Check sheet for the modelled part. Datum: model origin and axes. Units: mm. A direction names the side the tool comes from. Round coordinates to 2 decimals unless told otherwise and drop trailing zeros. Order: outer loops, then holes, each group sorted by start corner. A loop starts at its lowest first (then second) coordinate and runs counter-clockwise, first axis right, second up.
(1) Tool access check on faces 1 (the cylindrical face through (-42.3, -0.1, 8.5)), 2 (the cylindrical face through (-39.5, -0.1, 6.9)), 3 (the cylindrical face through (-35.14, 0.11, 3.9)), 4 (the flat face through (-1, 7.5, 2)). Record the directions out of +Z, -Z, +X, -X, +Y, -Y that give a thin tool (end or side, any length) a straight path to the whole face; none if there is none.
(2) Sectioned sample at A-A, the plane z = 1.5. Count the separate pieces of the cut face and the enclosed holes in it, and give its area (3 significant figures).
(3) Sectioned sample at C-C, the plane x = -10. Enter the section's corners in (y, z).
(4) Mould release check, pull along Y, two halves, no side actions. Record for faces 5 (the cylindrical face through (35.14, -0.11, 3.9)), 6 (the cylindrical face through (-39.6, 11.6, 6.4)), 7 (the flat face through (37.4, 0, 8)): released by +Y, released by -Y, zero draft, split by the parting line, or undercut.
(5) Thickness scan on probe 1 along Y at (x, z) = (-10, 0.9); probe 2 along X at (y, z) = (4, 2.35); probe 3 along Y at (x, z) = (-39.5, 3.25). Record the ranges inside material, lowest first.
(6) Depth check by flat-ended pin: pin 1 (3 mm diameter, centred on x = -7.5, z = 3.5, fed in from +Y); pin 2 (12 mm diameter, centred on x = -3, y = -2.5, fed in from +Z); pin 3 (2 mm diameter, centred on x = -9.5, z = 3, fed in from -Y). Enter the tip coordinate at first touch or a pass-through.
(7) Sectioned sample at B-B, the plane x = 39.5. Enter the section's corners in (y, z), and give its area (3 significant figures).
```python
from build123d import *

# Parameters (mm, degrees)
SKETCH1_W                                  = 86
SKETCH1_H                                  = 15
BOSS_EXTRUDE1_DEPTH                        = 3
SKETCH2_W                                  = 7
SKETCH2_H                                  = 15
BOSS_EXTRUDE2_DEPTH                        = 10
SKETCH5_R                                  = 4.5
CUT_EXTRUDE1_DEPTH                         = 88.299770905
SKETCH6_R                                  = 6.1
CUT_EXTRUDE4_DEPTH                         = 2.1
BOSS_EXTRUDE3_DEPTH                        = 13
SKETCH8_R                                  = 1.75
CUT_EXTRUDE5_DEPTH                         = 47.395689455
SKETCH9_R                                  = 1.75
CUT_EXTRUDE6_DEPTH                         = 46.6460294
MIRROR1_AT_THE_SECOND_PLANE_COPY_1_SKETC_R = 6.1
MIRROR1_AT_THE_SECOND_PLANE_COPY_1_DEPTH   = 2.1
MIRROR1_AT_THE_SECOND_PLANE_COPY_2_DEPTH   = 13
MIRROR1_AT_THE_SECOND_PLANE_COPY_3_SKETC_R = 1.75
MIRROR1_AT_THE_SECOND_PLANE_COPY_3_DEPTH   = 47.395689455
MIRROR1_AT_THE_SECOND_PLANE_COPY_4_SKETC_R = 1.75
MIRROR1_AT_THE_SECOND_PLANE_COPY_4_DEPTH   = 46.6460294
FILLET1_R                                  = 3


with BuildPart() as part:
    # Sketch1 → Boss-Extrude1 (new body)
    with BuildSketch(Plane.XY):
        Rectangle(SKETCH1_W, SKETCH1_H)
    extrude(amount=BOSS_EXTRUDE1_DEPTH)

    # Sketch2 → Boss-Extrude2 (add)
    with BuildSketch(Plane.XY.offset(3)):
        with Locations((-39.5, 0)):
            Rectangle(SKETCH2_W, SKETCH2_H)
        with Locations((39.5, 0)):
            Rectangle(SKETCH2_W, SKETCH2_H)
    extrude(amount=BOSS_EXTRUDE2_DEPTH)

    # Sketch5 → Cut-Extrude1 (cut, through all)
    with BuildSketch(Plane(origin=(43, 0, 0), x_dir=(0, 0, -1), z_dir=(1, 0, 0))):
        with Locations((-13, 0)):
            Circle(SKETCH5_R)
    extrude(amount=-CUT_EXTRUDE1_DEPTH, mode=Mode.SUBTRACT)

    # Sketch6 → Cut-Extrude4 (cut, symmetric)
    with BuildSketch(Plane(origin=(39.5, 0, 0), x_dir=(0, 0, -1), z_dir=(1, 0, 0))):
        with Locations((-13, 0)):
            Circle(SKETCH6_R)
    cut_extrude4 = extrude(amount=CUT_EXTRUDE4_DEPTH, both=True, mode=Mode.SUBTRACT)

    # Sketch7 → Boss-Extrude3 (add)
    with BuildSketch(Plane.XY):
        with BuildLine():
            Line((37.4, 6.1), (41.6, 6.1))
            Line((41.6, 6.1), (41.6, 4.5))
            Line((41.6, 4.5), (43, 4.5))
            Line((43, 4.5), (43, 8.1))
            ThreePointArc((43, 8.1), (39.5, 11.6), (36, 8.1))
            Line((36, 8.1), (36, 4.5))
            Line((36, 4.5), (37.4, 4.5))
            Line((37.4, 4.5), (37.4, 6.1))
        make_face()
    boss_extrude3 = extrude(amount=BOSS_EXTRUDE3_DEPTH)

    # Sketch8 → Cut-Extrude5 (cut, symmetric)
    with BuildSketch(Plane.XY.offset(13)):
        with Locations((39.5, 8.6)):
            Circle(SKETCH8_R)
    cut_extrude5 = extrude(amount=CUT_EXTRUDE5_DEPTH, both=True, mode=Mode.SUBTRACT)

    # Sketch9 → Cut-Extrude6 (cut, through all)
    with BuildSketch(Plane.XY.offset(3)):
        with Locations((-10, -4)):
            Circle(SKETCH9_R)
    cut_extrude6 = extrude(amount=-CUT_EXTRUDE6_DEPTH, mode=Mode.SUBTRACT)

    # Mirror1: Cut-Extrude4, Boss-Extrude3, Cut-Extrude5, Cut-Extrude6 across plane
    add(cut_extrude4.mirror(Plane(origin=(0, 0, 0), x_dir=(0, 0, 1), z_dir=(1, 0, 0))), mode=Mode.SUBTRACT)
    add(boss_extrude3.mirror(Plane(origin=(0, 0, 0), x_dir=(0, 0, 1), z_dir=(1, 0, 0))))
    add(cut_extrude5.mirror(Plane(origin=(0, 0, 0), x_dir=(0, 0, 1), z_dir=(1, 0, 0))), mode=Mode.SUBTRACT)
    add(cut_extrude6.mirror(Plane(origin=(0, 0, 0), x_dir=(0, 0, 1), z_dir=(1, 0, 0))), mode=Mode.SUBTRACT)

    # Mirror1 at the second plane: Cut-Extrude4, Boss-Extrude3, Cut-Extrude5, Cut-Extrude6 across plane
    add(cut_extrude4.mirror(Plane.ZX), mode=Mode.SUBTRACT)
    add(boss_extrude3.mirror(Plane.ZX))
    add(cut_extrude5.mirror(Plane.ZX), mode=Mode.SUBTRACT)
    add(cut_extrude6.mirror(Plane.ZX), mode=Mode.SUBTRACT)

    # Mirror1 at the second plane copy 1 sketc → Mirror1 at the second plane copy 1 (cut, symmetric)
    with BuildSketch(Plane(origin=(-39.5, 0, 0), x_dir=(0, 0, -1), z_dir=(-1, 0, 0))):
        with Locations((-13, 0)):
            Circle(MIRROR1_AT_THE_SECOND_PLANE_COPY_1_SKETC_R)
    extrude(amount=MIRROR1_AT_THE_SECOND_PLANE_COPY_1_DEPTH, both=True, mode=Mode.SUBTRACT)

    # Mirror1 at the second plane copy 2 sketc → Mirror1 at the second plane copy 2 (add)
    with BuildSketch(Plane(origin=(0, 0, 0), x_dir=(-1, 0, 0), z_dir=(0, 0, 1))):
        with BuildLine():
            Line((37.4, 6.1), (41.6, 6.1))
            Line((41.6, 6.1), (41.6, 4.5))
            Line((41.6, 4.5), (43, 4.5))
            Line((43, 4.5), (43, 8.1))
            ThreePointArc((43, 8.1), (39.5, 11.6), (36, 8.1))
            Line((36, 8.1), (36, 4.5))
            Line((36, 4.5), (37.4, 4.5))
            Line((37.4, 4.5), (37.4, 6.1))
        make_face()
    extrude(amount=MIRROR1_AT_THE_SECOND_PLANE_COPY_2_DEPTH)

    # Mirror1 at the second plane copy 3 sketc → Mirror1 at the second plane copy 3 (cut, symmetric)
    with BuildSketch(Plane(origin=(0, 0, 13), x_dir=(-1, 0, 0), z_dir=(0, 0, 1))):
        with Locations((39.5, 8.6)):
            Circle(MIRROR1_AT_THE_SECOND_PLANE_COPY_3_SKETC_R)
    extrude(amount=MIRROR1_AT_THE_SECOND_PLANE_COPY_3_DEPTH, both=True, mode=Mode.SUBTRACT)

    # Mirror1 at the second plane copy 4 sketc → Mirror1 at the second plane copy 4 (cut, through all)
    with BuildSketch(Plane(origin=(0, 0, 3), x_dir=(-1, 0, 0), z_dir=(0, 0, 1))):
        with Locations((-10, -4)):
            Circle(MIRROR1_AT_THE_SECOND_PLANE_COPY_4_SKETC_R)
    extrude(amount=-MIRROR1_AT_THE_SECOND_PLANE_COPY_4_DEPTH, mode=Mode.SUBTRACT)

    # Fillet1
    fillet1_edges = [part.edges().sort_by_distance(p)[0] for p in [
        (-36, 0, 3),
        (36, 0, 3),
    ]]
    fillet(fillet1_edges, radius=FILLET1_R)


solid = part.part
```
Derived:
1. face 1: +Z, +X, -X
1. face 2: +Z
1. face 3: +Z, +Y, -Y
1. face 4: +Z, -Z, +Y
2. separate pieces: 1
2. enclosed holes: 8
2. area: 1,310 mm2
3. outline: (-7.5, 0) - (-5.75, 0) - (-5.75, 3) - (-7.5, 3) - close; (-2.25, 0) - (2.25, 0) - (2.25, 3) - (-2.25, 3) - close; (5.75, 0) - (7.5, 0) - (7.5, 3) - (5.75, 3) - close
4. face 5: zero draft
4. face 6: released by +Y
4. face 7: undercut
5. probe 1: y = -7.5 to -5.75, -2.25 to 2.25, 5.75 to 7.5
5. probe 2: x = -43 to -11.75, -8.25 to 8.25, 11.75 to 43
5. probe 3: y = -11.6 to -10.35, -6.85 to 6.85, 10.35 to 11.6
6. pin 1: stops at y = 7.5
6. pin 2: stops at z = 3
6. pin 3: stops at y = -7.5
7. outline: (-11.6, 0) - (-10.35, 0) - (-10.35, 13) - (-11.6, 13) - close; (-6.85, 0) - (6.85, 0) - (6.85, 13) - (6.1, 13) arc R6.1 cw to (-6.1, 13) - (-6.85, 13) - close; (10.35, 0) - (11.6, 0) - (11.6, 13) - (10.35, 13) - close
7. area: 152 mm2
